from build123d import *

# Parameters (mm, degrees)
SKETCH1_W               = 40
SKETCH1_H               = 40
BOSS_EXTRUDE1_DEPTH     = 7.5
SKETCH2_R               = 19
CUT_EXTRUDE1_DEPTH      = 6.3
SKETCH3_W               = 25
SKETCH3_H               = 20
CUT_EXTRUDE2_DEPTH      = 6.3
SKETCH4_R               = 1.5
CUT_EXTRUDE3_DEPTH      = 30.261749777
SKETCH6_R               = 1.25
CUT_EXTRUDE5_DEPTH      = 29.977404991
SKETCH7_W               = 3
SKETCH7_H               = 6
BOSS_EXTRUDE2_DEPTH     = 6.3
FILLET1_R               = 10
FILLET2_R               = 10
SKETCH8_R               = 0.75
CUT_EXTRUDE6_DEPTH      = 30.261749777
BOSS_EXTRUDE3_DEPTH     = 5
FILLET3_R               = 1
CUT_EXTRUDE7_START      = -1
SKETCH10_W              = 3
SKETCH10_H              = 12
CUT_EXTRUDE7_DEPTH      = 2
CUT_EXTRUDE8_DEPTH      = 33.882366095
CUT_EXTRUDE8_DEPTH_BACK = 33.882366095
SKETCH11_W              = 5
SKETCH11_H              = 7.5
CUT_EXTRUDE9_START      = -5
SKETCH12_R              = 1.5
CUT_EXTRUDE9_DEPTH      = 5


with BuildPart() as part:
    # Sketch1 → Boss-Extrude1 (new body)
    with BuildSketch(Plane(origin=(0, 0, 0), x_dir=(1, 0, 0), z_dir=(0, 1, 0))):
        Rectangle(SKETCH1_W, SKETCH1_H)
    extrude(amount=BOSS_EXTRUDE1_DEPTH)

    # Sketch2 → Cut-Extrude1 (cut)
    with BuildSketch(Plane(origin=(0, 7.5, 0), x_dir=(1, 0, 0), z_dir=(0, 1, 0))):
        with Locations(Location((0, 0, 0), (0, 0, 270))):
            Circle(SKETCH2_R)
    extrude(amount=-CUT_EXTRUDE1_DEPTH, mode=Mode.SUBTRACT)

    # Sketch3 → Cut-Extrude2 (cut)
    with BuildSketch(Plane(origin=(0, 7.5, 0), x_dir=(1, 0, 0), z_dir=(0, 1, 0))):
        with Locations((-6.5, -10)):
            Rectangle(SKETCH3_W, SKETCH3_H)
    extrude(amount=-CUT_EXTRUDE2_DEPTH, mode=Mode.SUBTRACT)

    # Sketch4 → Cut-Extrude3 (cut, through all)
    with BuildSketch(Plane(origin=(0, 7.5, 0), x_dir=(1, 0, 0), z_dir=(0, 1, 0))):
        with Locations(Location((-16, 16, 0), (0, 0, 270))):
            Circle(SKETCH4_R)
        with Locations(Location((16, 16, 0), (0, 0, 270))):
            Circle(SKETCH4_R)
        with Locations(Location((16, -16, 0), (0, 0, 270))):
            Circle(SKETCH4_R)
    extrude(amount=-CUT_EXTRUDE3_DEPTH, mode=Mode.SUBTRACT)

    # Sketch6 → Cut-Extrude5 (cut, through all)
    with BuildSketch(Plane(origin=(0, 1.2, 0), x_dir=(1, 0, 0), z_dir=(0, 1, 0))):
        with Locations(Location((0, 0, 0), (0, 0, 270))):
            Circle(SKETCH6_R)
    extrude(amount=-CUT_EXTRUDE5_DEPTH, mode=Mode.SUBTRACT)

    # Sketch7 → Boss-Extrude2 (add)
    with BuildSketch(Plane(origin=(0, 1.2, 0), x_dir=(1, 0, 0), z_dir=(0, 1, 0))):
        with Locations((-17.5, -17)):
            Rectangle(SKETCH7_W, SKETCH7_H)
    extrude(amount=BOSS_EXTRUDE2_DEPTH)

    # Fillet1
    # the kernel refuses this fillet: 10 mm, written as the material it adds along each edge
    with BuildSketch(Plane(origin=(-19, 1.2, 14), x_dir=(0, 0, -1), z_dir=(0, 1, 0))) as fillet1_piece_1:
        with BuildLine():
            CenterArc((7.141428429, -10), FILLET1_R, 90, 45.572995999)
            Line((0, -3), (-0.142828569, -2.86))
            ThreePointArc((-0.142828569, -2.86), (-0.2, -1.5), (-0.2, 0))
            Line((-0.2, 0), (0, 0.2))
            Line((0, 0.2), (7.141428429, 0.2))
            Line((7.141428429, 0.2), (7.141428429, 0))
        make_face()
    extrude(amount=6.3)

    # Fillet2
    fillet2_edges = [part.edges().sort_by_distance(p)[0] for p in [
        (-16, 4.35, 14),
    ]]
    fillet(fillet2_edges, radius=FILLET2_R)

    # Sketch8 → Cut-Extrude6 (cut, through all)
    with BuildSketch(Plane(origin=(0, 7.5, 0), x_dir=(1, 0, 0), z_dir=(0, 1, 0))):
        with Locations(Location((-18, -17, 0), (0, 0, 270))):
            Circle(SKETCH8_R)
    extrude(amount=-CUT_EXTRUDE6_DEPTH, mode=Mode.SUBTRACT)

    # Sketch9 → Boss-Extrude3 (add)
    with BuildSketch(Plane.XY.offset(20)):
        Polygon((-18, 7.5), (-16, 7.5), (-16, 1.2), (6, 1.2), (6, 7.5), (8, 7.5), (8, 0), (-18, 0), align=None)
    extrude(amount=BOSS_EXTRUDE3_DEPTH)

    # Fillet3
    fillet3_edges = [part.edges().sort_by_distance(p)[0] for p in [
        (20, 3.75, 20),
        (-20, 3.75, 20),
        (-20, 3.75, -20),
        (20, 3.75, -20),
    ]]
    fillet(fillet3_edges, radius=FILLET3_R)

    # Sketch10 → Cut-Extrude7 (cut)
    with BuildSketch(Plane.XZ.offset(CUT_EXTRUDE7_START)):
        with Locations((1.5, -14)):
            Rectangle(SKETCH10_W, SKETCH10_H)
    extrude(amount=-CUT_EXTRUDE7_DEPTH, mode=Mode.SUBTRACT)

    # Sketch11 → Cut-Extrude8 (cut, two sides: drawn at the far end of the back side and taken through both)
    with BuildSketch(Plane(origin=(0, 0, 0), x_dir=(0, 0, -1), z_dir=(1, 0, 0)).offset(-CUT_EXTRUDE8_DEPTH_BACK)):
        with Locations((-22.5, 3.75)):
            Rectangle(SKETCH11_W, SKETCH11_H)
    extrude(amount=CUT_EXTRUDE8_DEPTH + CUT_EXTRUDE8_DEPTH_BACK, mode=Mode.SUBTRACT)

    # Sketch12 → Cut-Extrude9 (cut)
    # profile 1 of 2: a face of its own
    with BuildSketch(Plane.XZ.offset(CUT_EXTRUDE9_START)):
        with BuildLine():
            Line((20, -4), (19.595917942, -4))
            ThreePointArc((19.595917942, -4), (14.142135624, -14.142135624), (4, -19.595917942))
            Line((4, -19.595917942), (4, -20))
            Line((4, -20), (19, -20))
            ThreePointArc((19, -20), (19.707106781, -19.707106781), (20, -19))
            Line((20, -19), (20, -4))
        make_face()
        with Locations(Location((16, -16, 0), (0, 0, 90))):
            Circle(SKETCH12_R, mode=Mode.SUBTRACT)
    # profile 2 of 2: a face of its own
    with BuildSketch(Plane.XZ.offset(CUT_EXTRUDE9_START)):
        with BuildLine():
            Line((-4, -20), (-4, -19.595917942))
            ThreePointArc((-4, -19.595917942), (-14.142135624, -14.142135624), (-19.595917942, -4))
            Line((-19.595917942, -4), (-20, -4))
            Line((-20, -4), (-20, -19))
            ThreePointArc((-20, -19), (-19.707106781, -19.707106781), (-19, -20))
            Line((-19, -20), (-4, -20))
        make_face()
        with Locations(Location((-16, -16, 0), (0, 0, 90))):
            Circle(SKETCH12_R, mode=Mode.SUBTRACT)
    extrude(amount=CUT_EXTRUDE9_DEPTH, mode=Mode.SUBTRACT)


solid = part.part
Here's how the part is built. I have some questions about the finished solid (model axes, mm). A direction names the side the tool comes from. Round coordinates to 2 decimals unless told otherwise and drop trailing zeros. Loops run counter-clockwise (first coordinate to the right, second up) from the corner with the lowest first, then second, coordinate; pieces in that order, holes last. Notation, with made-up numbers: (-3, 81.25) - (26, 81.25) arc R32 cw to (26, 117.25) - close; hole circle Ø5 at (27, 35.5). An arc over 180 degrees is marked (long way). One line per question, with ' | ' between items. Start each with the question number.
Q1. We'd pull the mould along Z, two halves only. Please class faces 1 (the flat face through (4, 1, 20)), 2 (the cylindrical face through (-1.22, 0.61, -0.27)), 3 (the cylindrical face through (14.257, 2.535, -14.026)): +Z half, -Z half, draft (parallel to the pull), parting line (faces both ways), or undercut.
Q2. For faces 4 (the flat face through (1.5, 3, -19.5)), 5 (the flat face through (-14, 5, -16)), 6 (the cylindrical face through (11.581, 4.394, -15.062)), which set-ups out of +Z, -Z, +X, -X, +Y, -Y let a thin tool reach every point of the face, with its end or its side?
Q3. I want a section at C-C (z = 6). Write out the boundary of the cut face in (x, y), then the cut area to 3 significant figures.
Q4. Please list where these lines run through material, in increasing order: line 1 (X direction, y = 7, z = 0); line 2 (X direction, y = 5.75, z = 16); line 3 (X direction, y = 0.6, z = 0). Write a range as [from, to].
Q5. I want a section at B-B (x = -18). Write out the boundary of the cut face in (y, z), then the cut area to 3 significant figures.
Q6. Will these pins go through, and if not, where does the flat tip stop? pin 1 (2 mm diameter, centred on y = 1.5, z = -14.5, fed in from -X); pin 2 (2 mm diameter, centred on y = 2, z = -15.5, fed in from +X) (3 decimals); pin 3 (8 mm diameter, centred on x = -4, z = 11, fed in from +Y).
Q7. I want a section at A-A (y = 3.75). Write out the boundary of the cut face in (x, z).
Q8. I want a section at D-D (x = -3). Write out the boundary of the cut face in (y, z), then the cut area to 3 significant figures.
Response values:
1) face 1: +Z half | face 2: undercut | face 3: -Z half
2) face 4: +Z, -Z | face 5: -Z, -X, -Y | face 6: +Y
3) outline: (-20, 0) - (20, 0) - (20, 7.5) - (18.03, 7.5) - (18.03, 1.2) - (-19, 1.2) - (-19, 7.5) - (-20, 7.5) - close | area: 66.7 mm²
4) line 1: x = [-20, -19], [19, 20] | line 2: x = [-20, -16.1], [10.25, 14.5], [17.5, 20] | line 3: x = [-20, -1.25], [1.25, 20]
5) outline: (0, -8.72) - (5, -8.72) - (5, -20) - (7.5, -20) - (7.5, -6.08) - (1.2, -6.08) - (1.2, 11.22) - (7.5, 11.22) - (7.5, 16.25) - (0, 16.25) - close; (0, 17.75) - (7.5, 17.75) - (7.5, 20) - (0, 20) - close | area: 123 mm²
6) pin 1: stops at x = -14.76 | pin 2: stops at x = 13.775 | pin 3: stops at y = 1.2
7) outline: (-20, -4) - (-19.6, -4) arc R20 ccw to (-4, -19.6) - (-4, -20) - (4, -20) - (4, -19.6) arc R20 ccw to (19.6, -4) - (20, -4) - (20, 19) arc R1 ccw to (19, 20) - (6, 20) - (6, 18.03) arc R19 cw (long way) to (-19, 0) - (-19, 6.86) arc R10 cw to (-17.5, 12.13) arc R10 ccw to (-16, 17.39) - (-16, 20) - (-19, 20) arc R1 ccw to (-20, 19) - close; hole circle Ø1.5 at (-18, 17); hole circle Ø3 at (16, 16)
8) outline: (0, -20) - (7.5, -20) - (7.5, -18.76) - (1.2, -18.76) - (1.2, 20) - (0, 20) - close | area: 55.8 mm²
